Could you check a few things on this model? Use its own coordinates, in mm. A direction names the side the tool comes from. Round coordinates to 2 decimals unless told otherwise and drop trailing zeros. Loops run counter-clockwise (first coordinate to the right, second up) from the corner with the lowest first, then second, coordinate; pieces in that order, holes last.
from build123d import *

# Parameters (mm, degrees)
SKETCH1_R               = 14.125
SKETCH1_R_2             = 12.625
BOSS_EXTRUDE1_DEPTH     = 30
BOSS_EXTRUDE2_START     = 3
SKETCH2_R               = 14.125
BOSS_EXTRUDE2_DEPTH     = 3
BOSS_EXTRUDE3_START     = -25
BOSS_EXTRUDE3_OUTLINE_R = 4
BOSS_EXTRUDE3_DEPTH     = 50


# Read off the part's stored shape, not the designer's step: Boss-Extrude3
with BuildPart() as part:
    # Sketch1 → Boss-Extrude1 (new body)
    with BuildSketch(Plane(origin=(0, 0, 0), x_dir=(1, 0, 0), z_dir=(0, 1, 0))):
        with Locations(Location((0, 0, 0), (0, 0, 270))):
            Circle(SKETCH1_R)
        with Locations(Location((0, 0, 0), (0, 0, 270))):
            Circle(SKETCH1_R_2, mode=Mode.SUBTRACT)
    extrude(amount=BOSS_EXTRUDE1_DEPTH)

    # Sketch2 → Boss-Extrude2 (add)
    with BuildSketch(Plane(origin=(0, 0, 0), x_dir=(-1, 0, 0), z_dir=(0, -1, 0)).offset(BOSS_EXTRUDE2_START)):
        with Locations(Location((0, 0, 0), (0, 0, 90))):
            Circle(SKETCH2_R)
    extrude(amount=-BOSS_EXTRUDE2_DEPTH)

    # Boss-Extrude3 outline → Boss-Extrude3 (add)
    with BuildSketch(Plane.XY.offset(BOSS_EXTRUDE3_START)):
        with BuildLine():
            Line((14.125, -3), (14.125, -2))
            Line((14.125, -2), (-14.125, -2))
            Line((-14.125, -2), (-14.125, -3))
            ThreePointArc((-14.125, -3), (-11.408307596, -9.371443813), (-5, -12))
            Line((-5, -12), (5, -12))
            ThreePointArc((5, -12), (11.408307596, -9.371443813), (14.125, -3))
        make_face()
        with Locations((0, -7)):
            Circle(BOSS_EXTRUDE3_OUTLINE_R, mode=Mode.SUBTRACT)
    extrude(amount=BOSS_EXTRUDE3_DEPTH)


solid = part.part
Item 1: Will these pins go through, and if not, where does the flat tip stop? pin 1 (8 mm diameter, centred on x = 5, z = 2, fed in from +Y); pin 2 (1 mm diameter, centred on x = 9, y = 16, fed in from -Z); pin 3 (10 mm diameter, centred on x = 7.5, y = 14, fed in from -Z); pin 4 (6.5 mm diameter, centred on x = 0, y = -7, fed in from +Z) (3 decimals).
Results list:
pin 1: stops at y = 0
pin 2: stops at z = -11.28
pin 3: stops at z = -13.9
pin 4: passes through
Item 2: If we section it at D-D, the plane x = 3.25: Please give me the cut outline in (y, z).
Results list:
outline: (-12, -25) - (-9.33, -25) - (-9.33, 25) - (-12, 25) - close; (-4.67, -25) - (-2, -25) - (-2, -13.75) - (30, -13.75) - (30, -12.2) - (0, -12.2) - (0, 12.2) - (30, 12.2) - (30, 13.75) - (-2, 13.75) - (-2, 25) - (-4.67, 25) - close
Item 3: If we section it at B-B, the plane x = 0: Please give me the cut outline in (y, z) (3 decimals), then the cut area to 4 significant figures.
Results list:
outline: (-12, -25) - (-11, -25) - (-11, 25) - (-12, 25) - close; (-3, -25) - (-2, -25) - (-2, -14.125) - (30, -14.125) - (30, -12.625) - (0, -12.625) - (0, 12.625) - (30, 12.625) - (30, 14.125) - (-2, 14.125) - (-2, 25) - (-3, 25) - close
area: 246.5 mm2
Item 4: We'd pull the mould along Y, two halves only. Please class faces 1 (the cylindrical face through (-0.867, -10.905, -0.35)), 2 (the flat face through (0, -12, 0)), 3 (the flat face through (-0.2, -2.5, -25)): released by +Y, released by -Y, zero draft, split by the parting line, or undercut.
Results list:
face 1: undercut
face 2: released by -Y
face 3: zero draft
Item 5: If we section it at A-A, the plane z = 21: Please give me the cut outline in (x, y) (3 decimals).
Results list:
outline: (-14.125, -3) arc R9.126 ccw to (-5, -12) - (5, -12) arc R9.126 ccw to (14.125, -3) - (14.125, -2) - (-14.125, -2) - close; hole circle Ø8 at (0, -7)
Item 6: If I drill on line 1 along Y through (x, z) = (0, -7.5); line 2 along X through (y, z) = (9.5, 0) (3 decimals); line 3 along Y through (x, z) = (0, -15), over which ranges is the centre line in solid material (lowest first)?
Results list:
line 1: y = -12 to -11, -3 to 0
line 2: x = -14.125 to -12.625, 12.625 to 14.125
line 3: y = -12 to -11, -3 to -2
Item 7: If we section it at C-C, the plane y = -7: Please give me the cut outline in (x, z), then the cut area to 3 significant figures.
Results list:
outline: (-13.14, -25) - (-4, -25) - (-4, 25) - (-13.14, 25) - close; (4, -25) - (13.14, -25) - (13.14, 25) - (4, 25) - close
area: 914 mm2
Item 8: For faces 4 (the cylindrical face through (-7.68, 14.79, -10.02)), 5 (the flat face through (-7, 30, -11)), which set-ups out of +Z, -Z, +X, -X, +Y, -Y let a thin tool reach every point of the face, with its end or its side?
Results list:
face 4: +Y
face 5: +Z, -Z, +X, -X, +Y
